Can you work these out from the model? Positions are in its coordinate system, mm. Face numbers are marked on the shaded views. A direction names the side the tool comes from. Coordinates: 2 decimals unless noted, no trailing zeros. Order: outer loops, then holes, each group sorted by start corner. A loop starts at its lowest first (then second) coordinate and runs counter-clockwise, first axis right, second up. Notation, with made-up numbers: (59.5, -11) -> (78.5, -11) arc R24 cw to (78.5, 1) -> close; hole circle Ø5 at (-40, 76.5). An arc over 180 degrees is marked (long way). Answer in a Markdown table with one row per item.
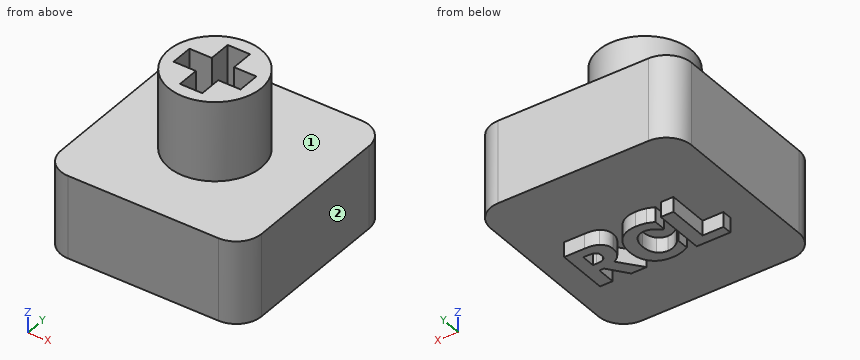
Autodesk Inventor part; units mm, degrees
ref_plane "Work Plane1" through (0, 0, 5) normal (0, 0, 1) x (1, 0, 0)
ref_plane "YZ Plane" through (0, 0, 0) normal (1, 0, 0) x (0, 1, 0)
ref_plane "XZ Plane" through (0, 0, 0) normal (0, 1, 0) x (-1, 0, 0)
sketch "Sketch1" plane through (0, 0, 0) normal (0, 0, 1) x (1, 0, 0)
  line L0 (14.6962, 12.74) -> (14.6962, 0) construction
  line L1 (10.61, 12.2) -> (1.53, 12.2)
  arc A0 (1.53, 12.2) -> (0, 10.67) centre (1.53, 10.67) ccw
  line L2 (0, 10.67) -> (0, 1.53)
  arc A1 (0, 1.53) -> (1.53, 0) centre (1.53, 1.53) ccw
  line L3 (1.53, 0) -> (10.61, 0)
  arc A2 (10.61, 0) -> (12.14, 1.53) centre (10.61, 1.53) ccw
  arc A3 (12.14, 10.67) -> (10.61, 12.2) centre (10.61, 10.67) ccw
  line L4 (12.14, 10.67) -> (12.14, 1.53)
  point P0 (0, 0)
  point P1 (0, 0)
  dimension "d10" = 12.74
ref_plane "Work Plane1" through (0, 0, 5) normal (0, 0, 1) x (1, 0, 0)
sketch "Sketch2" plane through (0, 0, 5) normal (0, 0, 1) x (1, 0, 0)
  line L0 (10.88, 12.74) -> (1.8, 12.74)
  line L1 (10.88, 12.74) -> (1.8, 12.74)
  arc A0 (1.8, 12.74) -> (0, 10.94) centre (1.8, 10.94) ccw
  line L2 (0, 10.94) -> (0, 1.8)
  arc A1 (0, 1.8) -> (1.8, 0) centre (1.8, 1.8) ccw
  line L3 (1.8, 0) -> (10.88, 0)
  arc A2 (10.88, 0) -> (12.68, 1.8) centre (10.88, 1.8) ccw
  line L4 (12.68, 1.8) -> (12.68, 10.94)
  arc A3 (12.68, 10.94) -> (10.88, 12.74) centre (10.88, 10.94) ccw
  circle A4 centre (6.34, 6.37) radius 2.8
  line L5 (5.665, 8.395) -> (7.015, 8.395)
  line L6 (7.015, 4.345) -> (5.665, 4.345)
  line L7 (5.665, 4.345) -> (7.015, 8.395) construction
  line L8 (5.665, 8.395) -> (7.015, 4.345) construction
  line L9 (8.365, 5.695) -> (8.365, 7.045)
  line L10 (4.315, 7.045) -> (4.315, 5.695)
  line L11 (4.315, 5.695) -> (8.365, 7.045) construction
  line L12 (8.365, 5.695) -> (4.315, 7.045) construction
  line L13 (4.315, 5.695) -> (5.665, 5.695)
  line L14 (7.015, 5.695) -> (8.365, 5.695)
  line L15 (5.665, 4.345) -> (5.665, 5.695)
  line L16 (5.665, 7.045) -> (5.665, 8.395)
  line L17 (8.365, 7.045) -> (7.015, 7.045)
  line L18 (5.665, 7.045) -> (4.315, 7.045)
  line L19 (7.015, 8.395) -> (7.015, 7.045)
  line L20 (7.015, 5.695) -> (7.015, 4.345)
  point P0 (0, 0)
  dimension "d3" = 5.6
  dimension "d4" = 4.05
  dimension "d5" = 1.35
  dimension "d6" = 4.05
  dimension "d7" = 1.35
extrude "Extrusion3" add sketch "Sketch1" along normal blind 5
sketch "Sketch3" plane through (0, 0, 5) normal (0, 0, 1) x (1, 0, 0)
  line L0 (10.61, 12.47) -> (1.53, 12.47)
  line L1 (10.61, 12.47) -> (1.53, 12.47)
  arc A0 (1.53, 12.47) -> (-0.27, 10.67) centre (1.53, 10.67) ccw
  line L2 (-0.27, 10.67) -> (-0.27, 1.53)
  arc A1 (-0.27, 1.53) -> (1.53, -0.27) centre (1.53, 1.53) ccw
  line L3 (1.53, -0.27) -> (10.61, -0.27)
  arc A2 (10.61, -0.27) -> (12.41, 1.53) centre (10.61, 1.53) ccw
  line L4 (12.41, 1.53) -> (12.41, 10.67)
  arc A3 (12.41, 10.67) -> (10.61, 12.47) centre (10.61, 10.67) ccw
  circle A4 centre (6.07, 6.1) radius 2.8
  line L5 (5.395, 8.125) -> (6.745, 8.125)
  line L6 (6.745, 4.075) -> (5.395, 4.075)
  line L7 (5.395, 4.075) -> (6.745, 8.125) construction
  line L8 (5.395, 8.125) -> (6.745, 4.075) construction
  line L9 (8.095, 5.425) -> (8.095, 6.775)
  line L10 (4.045, 6.775) -> (4.045, 5.425)
  line L11 (4.045, 5.425) -> (8.095, 6.775) construction
  line L12 (8.095, 5.425) -> (4.045, 6.775) construction
  line L13 (4.045, 5.425) -> (5.395, 5.425)
  line L14 (6.745, 5.425) -> (8.095, 5.425)
  line L15 (5.395, 4.075) -> (5.395, 5.425)
  line L16 (5.395, 6.775) -> (5.395, 8.125)
  line L17 (8.095, 6.775) -> (6.745, 6.775)
  line L18 (5.395, 6.775) -> (4.045, 6.775)
  line L19 (6.745, 8.125) -> (6.745, 6.775)
  line L20 (6.745, 5.425) -> (6.745, 4.075)
  line L21 (10.61, 12.2) -> (1.53, 12.2)
  line L22 (0, 10.67) -> (0, 1.53)
  point P0 (0, 0)
  point P1 (-0.27, -0.27)
  point P2 (6.07, 12.2)
  point P3 (0, 6.1)
  point P4 (6.07, 6.1)
  dimension "d14" = 5.6
  dimension "d15" = 4.05
  dimension "d16" = 1.35
  dimension "d17" = 4.05
  dimension "d18" = 1.35
extrude "Extrusion4" add sketch "Sketch3" along normal blind 4.8 contours A4
sketch "Sketch4" plane through (0, 0, 0) normal (0, 0, -1) x (-1, 0, 0)
  line L0 (-13.9436, 0) -> (-13.9436, 2.266)
  line L1 (-15.5559, 0) -> (-15.5559, 6.84)
  line L2 (-1.53, 0) -> (-10.61, 0)
  line L3 (-10.1927, 7.6843) -> (-1.9473, 7.6843) construction
  line L4 (-1.9473, 7.6843) -> (-1.9473, 4.5157) construction
  line L5 (-1.9473, 4.5157) -> (-10.1927, 4.5157) construction
  line L6 (-10.1927, 4.5157) -> (-10.1927, 7.6843) construction
  line L7 (-7.0587, 4.575) -> (-7.9905, 4.575)
  line L8 (-7.9905, 4.575) -> (-8.8382, 5.6947)
  line L9 (-8.8382, 5.6947) -> (-9.1151, 5.6947)
  line L10 (-9.1151, 5.6947) -> (-9.1151, 4.575)
  line L11 (-9.1151, 4.575) -> (-9.8763, 4.575)
  line L12 (-9.8763, 4.575) -> (-9.8763, 7.625)
  line L13 (-9.8763, 7.625) -> (-8.6504, 7.625)
  spline S0 degree 2 poles (-8.6504, 7.625) (-8.3958, 7.625) (-8.0201, 7.5607) (-7.8595, 7.4619) knots 0 0 0 1 2 2 2
  spline S1 degree 2 poles (-7.8595, 7.4619) (-7.6963, 7.3581) (-7.5035, 7.0343) (-7.5035, 6.7871) knots 0 0 0 1 2 2 2
  spline S2 degree 2 poles (-7.5035, 6.7871) (-7.5035, 6.4386) (-7.8199, 6.0011) (-8.0844, 5.8726) knots 0 0 0 1 2 2 2
  line L14 (-8.0844, 5.8726) -> (-7.0587, 4.575)
  spline S3 degree 2 poles (-8.2895, 6.6907) (-8.2895, 6.8069) (-8.3785, 6.9725) (-8.4798, 7.017) knots 0 0 0 1 2 2 2
  spline S4 degree 2 poles (-8.4798, 7.017) (-8.5515, 7.0466) (-8.727, 7.0639) (-8.858, 7.0639) knots 0 0 0 1 2 2 2
  line L15 (-8.858, 7.0639) -> (-9.1151, 7.0639)
  line L16 (-9.1151, 7.0639) -> (-9.1151, 6.2434)
  line L17 (-9.1151, 6.2434) -> (-8.8951, 6.2434)
  spline S5 degree 2 poles (-8.8951, 6.2434) (-8.7369, 6.2434) (-8.512, 6.2829) (-8.4354, 6.3447) knots 0 0 0 1 2 2 2
  spline S6 degree 2 poles (-8.4354, 6.3447) (-8.3612, 6.404) (-8.2895, 6.5622) (-8.2895, 6.6907) knots 0 0 0 1 2 2 2
  spline S7 degree 2 poles (-5.5164, 4.5157) (-6.2035, 4.5157) (-7.0092, 5.3462) (-7.0092, 6.0975) knots 0 0 0 1 2 2 2
  spline S8 degree 2 poles (-7.0092, 6.0975) (-7.0092, 6.8217) (-6.201, 7.6843) (-5.5139, 7.6843) knots 0 0 0 1 2 2 2
  spline S9 degree 2 poles (-5.5139, 7.6843) (-5.3335, 7.6843) (-5.0418, 7.6423) (-4.9083, 7.6077) knots 0 0 0 1 2 2 2
  spline S10 degree 2 poles (-4.9083, 7.6077) (-4.8045, 7.5756) (-4.5598, 7.4693) (-4.4832, 7.4297) knots 0 0 0 1 2 2 2
  line L18 (-4.4832, 7.4297) -> (-4.4832, 6.7031)
  line L19 (-4.4832, 6.7031) -> (-4.5598, 6.7031)
  spline S11 degree 2 poles (-4.5598, 6.7031) (-4.6167, 6.7525) (-4.7847, 6.8909) (-4.891, 6.9552) knots 0 0 0 1 2 2 2
  spline S12 degree 2 poles (-4.891, 6.9552) (-4.9973, 7.0219) (-5.2519, 7.1134) (-5.3928, 7.1134) knots 0 0 0 1 2 2 2
  spline S13 degree 2 poles (-5.3928, 7.1134) (-5.5584, 7.1134) (-5.8327, 7.0096) (-5.9588, 6.8786) knots 0 0 0 1 2 2 2
  spline S14 degree 2 poles (-5.9588, 6.8786) (-6.0725, 6.7624) (-6.2183, 6.3645) (-6.2183, 6.0951) knots 0 0 0 1 2 2 2
  spline S15 degree 2 poles (-6.2183, 6.0951) (-6.2183, 5.8108) (-6.0675, 5.4228) (-5.9439, 5.3041) knots 0 0 0 1 2 2 2
  spline S16 degree 2 poles (-5.9439, 5.3041) (-5.8253, 5.188) (-5.5337, 5.0866) (-5.3878, 5.0866) knots 0 0 0 1 2 2 2
  spline S17 degree 2 poles (-5.3878, 5.0866) (-5.2371, 5.0866) (-4.9627, 5.188) (-4.8688, 5.2498) knots 0 0 0 1 2 2 2
  spline S18 degree 2 poles (-4.8688, 5.2498) (-4.765, 5.3115) (-4.6093, 5.4425) (-4.5524, 5.4944) knots 0 0 0 1 2 2 2
  line L20 (-4.5524, 5.4944) -> (-4.4832, 5.4944)
  line L21 (-4.4832, 5.4944) -> (-4.4832, 4.7777)
  spline S19 degree 2 poles (-4.4832, 4.7777) (-4.5672, 4.7381) (-4.7872, 4.6393) (-4.9059, 4.6047) knots 0 0 0 1 2 2 2
  spline S20 degree 2 poles (-4.9059, 4.6047) (-5.0492, 4.5602) (-5.2988, 4.5157) (-5.5164, 4.5157) knots 0 0 0 1 2 2 2
  line L22 (-1.9967, 4.575) -> (-4.0309, 4.575)
  line L23 (-4.0309, 4.575) -> (-4.0309, 7.625)
  line L24 (-4.0309, 7.625) -> (-3.2647, 7.625)
  line L25 (-3.2647, 7.625) -> (-3.2647, 5.1558)
  line L26 (-3.2647, 5.1558) -> (-1.9967, 5.1558)
  line L27 (-1.9967, 5.1558) -> (-1.9967, 4.575)
  point P0 (0, 0)
  point P1 (-6.07, 0)
  point P2 (-6.07, 2.266)
  point P3 (-6.07, 6.1)
  point P4 (-6.07, 6.84)
  point P5 (-6.07, 4.5157)
  point P6 (-1.9473, 6.1)
  point P7 (-6.07, 6.1)
  dimension "d21" = 2.266
  dimension "d22" = 6.84
extrude "Extrusion5" add sketch "Sketch4" along normal blind 0.9
sketch "Sketch5" plane through (6.07, 6.1, 9.8) normal (0, 0, 1) x (1, 0, 0)
  circle A0 centre (0, 0) radius 2.8
  line L0 (-0.675, 0.675) -> (-0.675, 2.025)
  line L1 (-0.675, 2.025) -> (0.675, 2.025)
  line L2 (0.675, 2.025) -> (0.675, 0.675)
  line L3 (0.675, 0.675) -> (2.025, 0.675)
  line L4 (2.025, 0.675) -> (2.025, -0.675)
  line L5 (2.025, -0.675) -> (0.675, -0.675)
  line L6 (0.675, -0.675) -> (0.675, -2.025)
  line L7 (0.675, -2.025) -> (-0.675, -2.025)
  line L8 (-0.675, -2.025) -> (-0.675, -0.675)
  line L9 (-0.675, -0.675) -> (-2.025, -0.675)
  line L10 (-2.025, -0.675) -> (-2.025, 0.675)
  line L11 (-2.025, 0.675) -> (-0.675, 0.675)
  point P0 (-6.07, -6.1)
properties part number "IPC RCL key"
(1) Suppose I cut it at B-B (y = 2.75). Please give me the cut outline in (x, z), and give its area (3 significant figures).
Response values:
| item | result |
|---|---|
| outline | (0, 0) -> (12.14, 0) -> (12.14, 5) -> (0, 5) -> close |
| area | 60.7 mm2 |
(2) Will these pins go through, and if not, where does the flat tip stop? pin 1 Ø1.5 at (y, z) = (6, 8) entering from +X; pin 2 Ø1.5 at (y, z) = (6.5, 8) entering from -X; pin 3 Ø0.7 at (x, z) = (7.5, 8) entering from +Y.
Response values:
| item | result |
|---|---|
| pin 1 | x = 8.87 |
| pin 2 | x = 3.27 |
| pin 3 | y = 8.68 |
(3) Suppose I cut it at C-C (y = 4.25). Please give me the cut outline in (x, z) (3 decimals).
Response values:
| item | result |
|---|---|
| outline | (0, 0) -> (12.14, 0) -> (12.14, 5) -> (8.172, 5) -> (8.172, 9.8) -> (6.745, 9.8) -> (6.745, 5) -> (5.395, 5) -> (5.395, 9.8) -> (3.968, 9.8) -> (3.968, 5) -> (0, 5) -> close |
(4) On a 3-axis mill with a long thin cutter (end or side, diameter ignored), from which of +Z, -Z, +X, -X, +Y, -Y can I reach the whole of each face in a straight line? I mean the marked faces 1 and 2. Say none if no direction works.
Response values:
| item | result |
|---|---|
| face 1 | +Z |
| face 2 | +Z, -Z, +X, +Y, -Y |
(5) Suppose I cut it at A-A (z = 7.25). Please give me the cut outline in (x, y) (3 decimals).
Response values:
| item | result |
|---|---|
| outline | circle Ø5.6 at (6.07, 6.1); hole (4.045, 5.425) -> (5.395, 5.425) -> (5.395, 4.075) -> (6.745, 4.075) -> (6.745, 5.425) -> (8.095, 5.425) -> (8.095, 6.775) -> (6.745, 6.775) -> (6.745, 8.125) -> (5.395, 8.125) -> (5.395, 6.775) -> (4.045, 6.775) -> close |
(6) I need wall thicknesses on line 1 (Z direction, x = 5, y = 5.5); line 2 (Z direction, x = 4, y = 4.5); line 3 (Y direction, x = 5.5, z = 7.75) (3 decimals). Which ranges of each line are inside material? Lowest first, please. Write a range as [from, to].
Response values:
| item | result |
|---|---|
| line 1 | [0, 5] |
| line 2 | [0, 9.8] |
| line 3 | [3.359, 4.075], [8.125, 8.841] |
